Can you work these out from the model? Positions are in its coordinate system, mm. Face numbers are marked on the shaded views. A direction names the side the tool comes from. Coordinates: 2 decimals unless noted, no trailing zeros. Loops run counter-clockwise (first coordinate to the right, second up) from the corner with the lowest first, then second, coordinate; pieces in that order, holes last. Notation, with made-up numbers: (-17, 17.5) -> (24, 17.5) arc R20 ccw to (24, 51.5) -> close; hole circle Ø3 at (-22, 66). An arc over 180 degrees is marked (long way). Use one line per item in the form item = value. Start each with the question number.
(1) Imagine slicing it at A-A (y = 0). List the corners of the cut face in (x, z) for me.
(2) I need wall thicknesses on line 1 (Z direction, x = -1.1, y = 0.2); line 2 (Z direction, x = 1.1, y = 1.65); line 3 (Y direction, x = -0.1, z = 8.75). Which ranges of each line are inside material? Lowest first, please. Write a range as [from, to].
(3) On a 3-axis mill with a long thin cutter (end or side, diameter ignored), from which of +Z, -Z, +X, -X, +Y, -Y can I reach the whole of each face in a straight line? I mean the marked faces 4 and 5. Say none if no direction works.
(4) I'm going to push flat-ended pins straight in: pin 1 (1.5 mm diameter, centred on x = -2, z = 4, fed in from -Y); pin 2 (3 mm diameter, centred on y = -1.5, z = 4.5, fed in from +X); pin 3 (1.3 mm diameter, centred on x = 0, y = 0.5, fed in from -Z). Where does each tip first touch, or does it pass through?
(5) Imagine slicing it at B-B (z = 5.5). List the corners of the cut face in (x, y) for me, plus the area to 3 significant figures.
(6) Imagine slicing it at C-C (z = -0.5). List the corners of the cut face in (x, y) for me, plus the area to 3 significant figures.
(7) Thinking about a two-plate mould opening in X: for the marked faces 1, 2 and 3, which applies, released by +X, released by -X, zero draft, split by the parting line, or undercut?
Autodesk Inventor part; units mm, degrees
ref_plane "YZ Plane" through (0, 0, 0) normal (1, 0, 0) x (0, 1, 0)
ref_plane "XZ Plane" through (0, 0, 0) normal (0, 1, 0) x (-1, 0, 0)
ref_plane "XY Plane" through (0, 0, 0) normal (0, 0, 1) x (1, 0, 0)
sketch "스케치1" plane through (0, 0, 0) normal (0, 0, 1) x (1, 0, 0)
  circle A0 centre (0, 0) radius 1.5
  dimension "d0" = 3
extrude "돌출1" add sketch "스케치1" along normal blind 15
chamfer "모따기1" distance 0.2 angle 45 1 edges at (-1.5, 0, 15)
sketch "스케치2" plane through (0, 0, 0) normal (0, 0, -1) x (-1, 0, 0)
  circle A0 centre (0, 0) radius 2.75
  dimension "d6" = 5.5
extrude "돌출2" add sketch "스케치2" along normal blind 3
fillet "모깎기1" radius 0.2 2 edges at (2.75, 0, 0) (2.75, 0, -3)
sketch "스케치3" plane through (0, 0, -3) normal (0, 0, -1) x (-1, 0, 0)
  line L0 (0, 1.4434) -> (1.25, 0.7217)
  line L1 (1.25, 0.7217) -> (1.25, -0.7217)
  line L2 (1.25, -0.7217) -> (0, -1.4434)
  line L3 (0, -1.4434) -> (-1.25, -0.7217)
  line L4 (-1.25, -0.7217) -> (-1.25, 0.7217)
  line L5 (-1.25, 0.7217) -> (0, 1.4434)
  point P0 (0, 0)
  point P1 (0, 0)
  point P2 (-1.25, 0)
  dimension "d10" = 2.5
extrude "돌출3" cut sketch "스케치3" against normal blind 1.5
thread "스레드1"
properties part number "육각렌치볼트 m3 15mm"
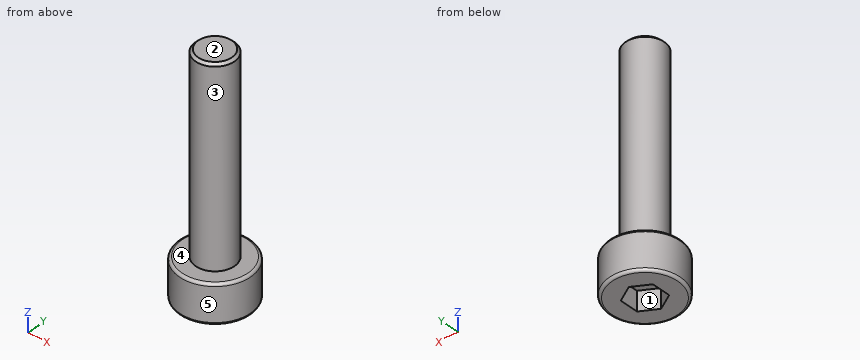
Worked out:
q1.outline = (-2.75, -2.8) arc R0.2 ccw to (-2.55, -3) -> (-1.25, -3) -> (-1.25, -1.5) -> (1.25, -1.5) -> (1.25, -3) -> (2.55, -3) arc R0.2 ccw to (2.75, -2.8) -> (2.75, -0.2) arc R0.2 ccw to (2.55, 0) -> (1.5, 0) -> (1.5, 14.8) -> (1.3, 15) -> (-1.3, 15) -> (-1.5, 14.8) -> (-1.5, 0) -> (-2.55, 0) arc R0.2 ccw to (-2.75, -0.2) -> close
q2.line_1 = [-1.5, 15]
q2.line_2 = [-3, 0]
q2.line_3 = [-1.5, 1.5]
q3.face_4 = +Z
q3.face_5 = +Z, -Z
q4.pin_1 = -0.83
q4.pin_2 = 1.5
q4.pin_3 = -1.5
q5.outline = circle Ø3 at (0, 0)
q5.area = 7.07 mm2
q6.outline = circle Ø5.5 at (0, 0)
q6.area = 23.8 mm2
q7.face_1 = undercut
q7.face_2 = zero draft
q7.face_3 = split by the parting line
